For this review, take the finished solid that the model builds, in its own axes (mm). Coordinates: 2 decimals unless noted, no trailing zeros. Loops run counter-clockwise (first coordinate to the right, second up) from the corner with the lowest first, then second, coordinate; pieces in that order, holes last. Notation, with made-up numbers: M -18.5,2 L 23.5,2 A16 ccw 23.5,25 Z; hole C 22.5,-2 d5. An arc over 180 degrees is marked long. Answer as a JSON object with one key per item and string values. Group by question number.
Item 1: Add section A-A (y = 118.5). State the section outline as (x, z) points.
Item 2: Insertion check: pin 1 (0.5 mm diameter, centred on y = 7, z = 0.5, fed in from +X); pin 2 (5 mm diameter, centred on x = 396.748, y = 142.24, fed in from +Z). Each pin has a flat end and moves straight along its axis. Give the tip position at first contact, or say it passes through.
Item 3: Add section B-B (z = 1.15). Count the separate pieces of the cut face and the enclosed holes in it, then the cut area to 3 significant figures.
Item 4: Wall thickness on L1, parallel to X at y = 113, z = 0.2; L2, parallel to X at y = 5.08, z = 0.05; L3, parallel to Y at x = 4.5, z = 1.5: over which ranges is each line inside the solid? List them lowest first. Write a range as from..to.
from build123d import *

# Parameters (mm, degrees)
MODEL_R                                       = 1.8288
BOSS_EXTRUDE2_DEPTH                           = 1.5875
CSK_FOR_6_FLAT_HEAD_MACHINE_SCREW2_AT_2_COUNT = 2
CSK_FOR_6_FLAT_HEAD_MACHINE_SCREW2_AT_2_PITCH = 79.248
CSK_FOR_6_FLAT_HEAD_MACHINE_SCREW2_AT_3_COUNT = 2
CSK_FOR_6_FLAT_HEAD_MACHINE_SCREW2_AT_3_PITCH = 157.48
CSK_FOR_6_FLAT_HEAD_MACHINE_SCREW2_AT_4_COUNT = 2
CSK_FOR_6_FLAT_HEAD_MACHINE_SCREW2_AT_4_PITCH = 235.712
CSK_FOR_6_FLAT_HEAD_MACHINE_SCREW2_AT_5_COUNT = 2
CSK_FOR_6_FLAT_HEAD_MACHINE_SCREW2_AT_5_PITCH = 313.944
CSK_FOR_6_FLAT_HEAD_MACHINE_SCREW2_AT_6_COUNT = 2
CSK_FOR_6_FLAT_HEAD_MACHINE_SCREW2_AT_6_PITCH = 391.668
CSK_FOR_6_FLAT_HEAD_MACHINE_SCREW2_AT_7_COUNT = 2
CSK_FOR_6_FLAT_HEAD_MACHINE_SCREW2_AT_7_PITCH = 447.04
CSK_FOR_6_FLAT_HEAD_MACHINE_SCREW2_AT_8_COUNT = 2
CSK_FOR_6_FLAT_HEAD_MACHINE_SCREW2_AT_8_PITCH = 451.707775558
CSK_FOR_6_FLAT_HEAD_MACHINE_SCREW2_AT_9_COUNT = 2
CSK_FOR_6_FLAT_HEAD_MACHINE_SCREW2_AT_9_PITCH = 403.385588022
CSK_FOR_6_FLAT_HEAD_MACHINE_SCREW2_AT_1_COUNT = 2
CSK_FOR_6_FLAT_HEAD_MACHINE_SCREW2_AT_1_PITCH = 425.043329819
CSK_FOR_6_FLAT_HEAD_MACHINE_SCREW2_2_COUNT    = 2
CSK_FOR_6_FLAT_HEAD_MACHINE_SCREW2_2_PITCH    = 456.08131361
CSK_FOR_6_FLAT_HEAD_MACHINE_SCREW2_3_COUNT    = 2
CSK_FOR_6_FLAT_HEAD_MACHINE_SCREW2_3_PITCH    = 331.913376266
CSK_FOR_6_FLAT_HEAD_MACHINE_SCREW2_4_COUNT    = 2
CSK_FOR_6_FLAT_HEAD_MACHINE_SCREW2_4_PITCH    = 287.78143954
CSK_FOR_6_FLAT_HEAD_MACHINE_SCREW2_5_COUNT    = 2
CSK_FOR_6_FLAT_HEAD_MACHINE_SCREW2_5_PITCH    = 254.708180756
CSK_FOR_6_FLAT_HEAD_MACHINE_SCREW2_6_COUNT    = 2
CSK_FOR_6_FLAT_HEAD_MACHINE_SCREW2_6_PITCH    = 124.885371057
CSK_FOR_6_FLAT_HEAD_MACHINE_SCREW2_7_COUNT    = 2
CSK_FOR_6_FLAT_HEAD_MACHINE_SCREW2_7_PITCH    = 183.134528432
CSK_FOR_6_FLAT_HEAD_MACHINE_SCREW2_8_COUNT    = 2
CSK_FOR_6_FLAT_HEAD_MACHINE_SCREW2_8_PITCH    = 246.752077811


with BuildPart() as part:
    # Model → Boss-Extrude2 (new body)
    with BuildSketch(Plane.XY):
        with BuildLine():
            Line((-25.251805612, 0), (0.148194388, 0))
            Line((0.148194388, 0), (415.374694388, 0))
            ThreePointArc((415.374694388, 0), (415.393293107, 0.044901281), (415.438194388, 0.0635))
            Line((415.438194388, 0.0635), (415.438194388, 10.0965))
            ThreePointArc((415.438194388, 10.0965), (415.393293107, 10.204901281), (415.501694388, 10.16))
            Line((415.501694388, 10.16), (457.284694388, 10.16))
            ThreePointArc((457.284694388, 10.16), (457.303293107, 10.204901281), (457.348194388, 10.2235))
            Line((457.348194388, 10.2235), (457.348194388, 243.7765))
            ThreePointArc((457.348194388, 243.7765), (457.303293107, 243.795098719), (457.284694388, 243.84))
            Line((457.284694388, 243.84), (0.211694388, 243.84))
            ThreePointArc((0.211694388, 243.84), (0.193095668, 243.795098719), (0.148194388, 243.7765))
            ThreePointArc((0.148194388, 243.7765), (0.103293107, 243.795098719), (0.084694388, 243.84))
            Line((0.084694388, 243.84), (-25.251805612, 243.84))
            ThreePointArc((-25.251805612, 243.84), (-29.741933673, 241.980128061), (-31.601805612, 237.49))
            Line((-31.601805612, 237.49), (-31.601805612, 6.35))
            ThreePointArc((-31.601805612, 6.35), (-29.741933673, 1.859871939), (-25.251805612, 0))
        make_face()
        with Locations((84.328, 5.08)):
            Circle(MODEL_R, mode=Mode.SUBTRACT)
        with BuildLine():
            Line((-18.901805612, 68.58), (-6.201805612, 68.58))
            ThreePointArc((-6.201805612, 68.58), (-1.711677552, 66.720128061), (0.148194388, 62.23))
            Line((0.148194388, 62.23), (0.148194388, 16.51))
            ThreePointArc((0.148194388, 16.51), (-1.711677552, 12.019871939), (-6.201805612, 10.16))
            Line((-6.201805612, 10.16), (-18.901805612, 10.16))
            ThreePointArc((-18.901805612, 10.16), (-23.391933673, 12.019871939), (-25.251805612, 16.51))
            Line((-25.251805612, 16.51), (-25.251805612, 62.23))
            ThreePointArc((-25.251805612, 62.23), (-23.391933673, 66.720128061), (-18.901805612, 68.58))
        make_face(mode=Mode.SUBTRACT)
        with Locations((84.328, 73.66)):
            Circle(MODEL_R, mode=Mode.SUBTRACT)
        with BuildLine():
            Line((-18.901805612, 137.16), (-6.201805612, 137.16))
            ThreePointArc((-6.201805612, 137.16), (-1.711677552, 135.300128061), (0.148194388, 130.81))
            Line((0.148194388, 130.81), (0.148194388, 85.09))
            ThreePointArc((0.148194388, 85.09), (-1.711677552, 80.599871939), (-6.201805612, 78.74))
            Line((-6.201805612, 78.74), (-18.901805612, 78.74))
            ThreePointArc((-18.901805612, 78.74), (-23.391933673, 80.599871939), (-25.251805612, 85.09))
            Line((-25.251805612, 85.09), (-25.251805612, 130.81))
            ThreePointArc((-25.251805612, 130.81), (-23.391933673, 135.300128061), (-18.901805612, 137.16))
        make_face(mode=Mode.SUBTRACT)
        with Locations((240.792, 5.08)):
            Circle(MODEL_R, mode=Mode.SUBTRACT)
        with Locations((396.748, 5.08)):
            Circle(MODEL_R, mode=Mode.SUBTRACT)
        with Locations((240.792, 73.66)):
            Circle(MODEL_R, mode=Mode.SUBTRACT)
        with Locations((396.748, 73.66)):
            Circle(MODEL_R, mode=Mode.SUBTRACT)
        with Locations((84.328, 142.24)):
            Circle(MODEL_R, mode=Mode.SUBTRACT)
        with BuildLine():
            ThreePointArc((-6.201805612, 233.68), (-1.711677552, 231.820128061), (0.148194388, 227.33))
            Line((0.148194388, 227.33), (0.148194388, 153.67))
            ThreePointArc((0.148194388, 153.67), (-1.711677552, 149.179871939), (-6.201805612, 147.32))
            Line((-6.201805612, 147.32), (-18.901805612, 147.32))
            ThreePointArc((-18.901805612, 147.32), (-23.391933673, 149.179871939), (-25.251805612, 153.67))
            Line((-25.251805612, 153.67), (-25.251805612, 227.33))
            ThreePointArc((-25.251805612, 227.33), (-23.391933673, 231.820128061), (-18.901805612, 233.68))
            Line((-18.901805612, 233.68), (-6.201805612, 233.68))
        make_face(mode=Mode.SUBTRACT)
        with Locations((5.08, 238.76)):
            Circle(MODEL_R, mode=Mode.SUBTRACT)
        with Locations((84.328, 238.76)):
            Circle(MODEL_R, mode=Mode.SUBTRACT)
        with Locations((162.56, 238.76)):
            Circle(MODEL_R, mode=Mode.SUBTRACT)
        with Locations((240.792, 142.24)):
            Circle(MODEL_R, mode=Mode.SUBTRACT)
        with Locations((396.748, 142.24)):
            Circle(MODEL_R, mode=Mode.SUBTRACT)
        with Locations((452.12, 173.99)):
            Circle(MODEL_R, mode=Mode.SUBTRACT)
        with Locations((240.792, 238.76)):
            Circle(MODEL_R, mode=Mode.SUBTRACT)
        with Locations((319.024, 238.76)):
            Circle(MODEL_R, mode=Mode.SUBTRACT)
        with Locations((396.748, 238.76)):
            Circle(MODEL_R, mode=Mode.SUBTRACT)
        with Locations((452.12, 238.76)):
            Circle(MODEL_R, mode=Mode.SUBTRACT)
    extrude(amount=BOSS_EXTRUDE2_DEPTH)

    # Sketch4 → CSK for #6 Flat Head Machine Screw2 (revolve, cut)
    with BuildSketch(Plane(origin=(5.08, 238.76, 1.5875), x_dir=(0, -1, 0), z_dir=(1, 0, 0))):
        Polygon((0, 0), (0, 1.5875), (1.8288, 1.5875), (1.8288, 1.519406592), (3.1496, 0), align=None)
    csk_for_6_flat_head_machine_screw2 = revolve(axis=Axis((5.08, 238.76, 7.9375), (0, 0, -1)), mode=Mode.SUBTRACT)

    # CSK for #6 Flat Head Machine Screw2 at 2: CSK for #6 Flat Head Machine Screw2 ×2
    with Locations(*[(i * CSK_FOR_6_FLAT_HEAD_MACHINE_SCREW2_AT_2_PITCH, 0, 0) for i in range(1, CSK_FOR_6_FLAT_HEAD_MACHINE_SCREW2_AT_2_COUNT)]):
        add(csk_for_6_flat_head_machine_screw2, mode=Mode.SUBTRACT)

    # CSK for #6 Flat Head Machine Screw2 at 3: CSK for #6 Flat Head Machine Screw2 ×2
    with Locations(*[(i * CSK_FOR_6_FLAT_HEAD_MACHINE_SCREW2_AT_3_PITCH, 0, 0) for i in range(1, CSK_FOR_6_FLAT_HEAD_MACHINE_SCREW2_AT_3_COUNT)]):
        add(csk_for_6_flat_head_machine_screw2, mode=Mode.SUBTRACT)

    # CSK for #6 Flat Head Machine Screw2 at 4: CSK for #6 Flat Head Machine Screw2 ×2
    with Locations(*[(i * CSK_FOR_6_FLAT_HEAD_MACHINE_SCREW2_AT_4_PITCH, 0, 0) for i in range(1, CSK_FOR_6_FLAT_HEAD_MACHINE_SCREW2_AT_4_COUNT)]):
        add(csk_for_6_flat_head_machine_screw2, mode=Mode.SUBTRACT)

    # CSK for #6 Flat Head Machine Screw2 at 5: CSK for #6 Flat Head Machine Screw2 ×2
    with Locations(*[(i * CSK_FOR_6_FLAT_HEAD_MACHINE_SCREW2_AT_5_PITCH, 0, 0) for i in range(1, CSK_FOR_6_FLAT_HEAD_MACHINE_SCREW2_AT_5_COUNT)]):
        add(csk_for_6_flat_head_machine_screw2, mode=Mode.SUBTRACT)

    # CSK for #6 Flat Head Machine Screw2 at 6: CSK for #6 Flat Head Machine Screw2 ×2
    with Locations(*[(i * CSK_FOR_6_FLAT_HEAD_MACHINE_SCREW2_AT_6_PITCH, 0, 0) for i in range(1, CSK_FOR_6_FLAT_HEAD_MACHINE_SCREW2_AT_6_COUNT)]):
        add(csk_for_6_flat_head_machine_screw2, mode=Mode.SUBTRACT)

    # CSK for #6 Flat Head Machine Screw2 at 7: CSK for #6 Flat Head Machine Screw2 ×2
    with Locations(*[(i * CSK_FOR_6_FLAT_HEAD_MACHINE_SCREW2_AT_7_PITCH, 0, 0) for i in range(1, CSK_FOR_6_FLAT_HEAD_MACHINE_SCREW2_AT_7_COUNT)]):
        add(csk_for_6_flat_head_machine_screw2, mode=Mode.SUBTRACT)

    # CSK for #6 Flat Head Machine Screw2 at 8: CSK for #6 Flat Head Machine Screw2 ×2
    with Locations(*[Vector(0.989666382, -0.143389163, 0) * (i * CSK_FOR_6_FLAT_HEAD_MACHINE_SCREW2_AT_8_PITCH) for i in range(1, CSK_FOR_6_FLAT_HEAD_MACHINE_SCREW2_AT_8_COUNT)]):
        add(csk_for_6_flat_head_machine_screw2, mode=Mode.SUBTRACT)

    # CSK for #6 Flat Head Machine Screw2 at 9: CSK for #6 Flat Head Machine Screw2 ×2
    with Locations(*[Vector(0.970951892, -0.239274785, 0) * (i * CSK_FOR_6_FLAT_HEAD_MACHINE_SCREW2_AT_9_PITCH) for i in range(1, CSK_FOR_6_FLAT_HEAD_MACHINE_SCREW2_AT_9_COUNT)]):
        add(csk_for_6_flat_head_machine_screw2, mode=Mode.SUBTRACT)

    # CSK for #6 Flat Head Machine Screw2 at 1: CSK for #6 Flat Head Machine Screw2 ×2
    with Locations(*[Vector(0.921477818, -0.388430987, 0) * (i * CSK_FOR_6_FLAT_HEAD_MACHINE_SCREW2_AT_1_PITCH) for i in range(1, CSK_FOR_6_FLAT_HEAD_MACHINE_SCREW2_AT_1_COUNT)]):
        add(csk_for_6_flat_head_machine_screw2, mode=Mode.SUBTRACT)

    # CSK for #6 Flat Head Machine Screw2  2: CSK for #6 Flat Head Machine Screw2 ×2
    with Locations(*[Vector(0.858767918, -0.512364776, 0) * (i * CSK_FOR_6_FLAT_HEAD_MACHINE_SCREW2_2_PITCH) for i in range(1, CSK_FOR_6_FLAT_HEAD_MACHINE_SCREW2_2_COUNT)]):
        add(csk_for_6_flat_head_machine_screw2, mode=Mode.SUBTRACT)

    # CSK for #6 Flat Head Machine Screw2  3: CSK for #6 Flat Head Machine Screw2 ×2
    with Locations(*[Vector(0.710161195, -0.704039116, 0) * (i * CSK_FOR_6_FLAT_HEAD_MACHINE_SCREW2_3_PITCH) for i in range(1, CSK_FOR_6_FLAT_HEAD_MACHINE_SCREW2_3_COUNT)]):
        add(csk_for_6_flat_head_machine_screw2, mode=Mode.SUBTRACT)

    # CSK for #6 Flat Head Machine Screw2  4: CSK for #6 Flat Head Machine Screw2 ×2
    with Locations(*[Vector(0.819066026, -0.573699264, 0) * (i * CSK_FOR_6_FLAT_HEAD_MACHINE_SCREW2_4_PITCH) for i in range(1, CSK_FOR_6_FLAT_HEAD_MACHINE_SCREW2_4_COUNT)]):
        add(csk_for_6_flat_head_machine_screw2, mode=Mode.SUBTRACT)

    # CSK for #6 Flat Head Machine Screw2  5: CSK for #6 Flat Head Machine Screw2 ×2
    with Locations(*[Vector(0.925419825, -0.378943463, 0) * (i * CSK_FOR_6_FLAT_HEAD_MACHINE_SCREW2_5_PITCH) for i in range(1, CSK_FOR_6_FLAT_HEAD_MACHINE_SCREW2_5_COUNT)]):
        add(csk_for_6_flat_head_machine_screw2, mode=Mode.SUBTRACT)

    # CSK for #6 Flat Head Machine Screw2  6: CSK for #6 Flat Head Machine Screw2 ×2
    with Locations(*[Vector(0.634565917, -0.772868745, 0) * (i * CSK_FOR_6_FLAT_HEAD_MACHINE_SCREW2_6_PITCH) for i in range(1, CSK_FOR_6_FLAT_HEAD_MACHINE_SCREW2_6_COUNT)]):
        add(csk_for_6_flat_head_machine_screw2, mode=Mode.SUBTRACT)

    # CSK for #6 Flat Head Machine Screw2  7: CSK for #6 Flat Head Machine Screw2 ×2
    with Locations(*[Vector(0.432731068, -0.901523057, 0) * (i * CSK_FOR_6_FLAT_HEAD_MACHINE_SCREW2_7_PITCH) for i in range(1, CSK_FOR_6_FLAT_HEAD_MACHINE_SCREW2_7_COUNT)]):
        add(csk_for_6_flat_head_machine_screw2, mode=Mode.SUBTRACT)

    # CSK for #6 Flat Head Machine Screw2  8: CSK for #6 Flat Head Machine Screw2 ×2
    with Locations(*[Vector(0.321164469, -0.947023434, 0) * (i * CSK_FOR_6_FLAT_HEAD_MACHINE_SCREW2_8_PITCH) for i in range(1, CSK_FOR_6_FLAT_HEAD_MACHINE_SCREW2_8_COUNT)]):
        add(csk_for_6_flat_head_machine_screw2, mode=Mode.SUBTRACT)


solid = part.part
From the geometry:
{
 "1": {"outline": "M -31.6,0 L -25.25,0 L -25.25,1.59 L -31.6,1.59 Z; M 0.15,0 L 457.35,0 L 457.35,1.59 L 0.15,1.59 Z"},
 "2": {"pin 1": "stops at x = 415.44", "pin 2": "stops at z = 0.84"},
 "3": {"separate pieces": "1", "enclosed holes": "20", "area": "113,000 mm²"},
 "4": {"L1": "x = -31.6..-25.25, 0.15..457.35", "L2": "x = -31.47..82.5, 86.16..238.96, 242.62..394.92, 398.58..415.44", "L3": "y = 0..235.74, 241.78..243.84"}
}
